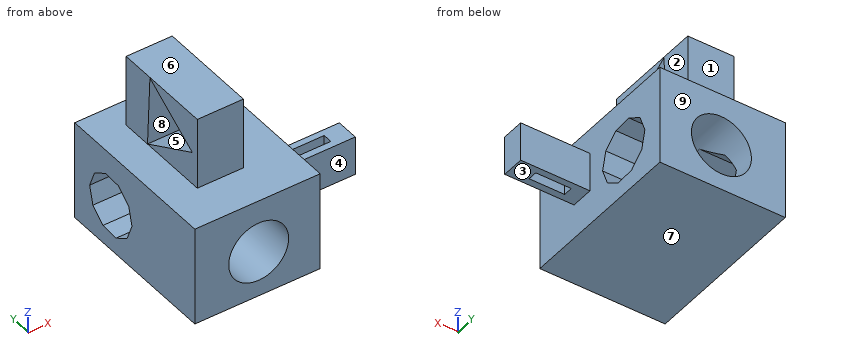
```python
from build123d import *

# Parameters (mm, degrees)
F0_W      = 94.7674
F0_H      = 75.057
F1_DEPTH  = 64.262
F2_W      = 34.8323993385
F2_H      = 76.1452428997
F3_DEPTH  = 92.202
F4_W      = 17.0815913007
F4_H      = 29.5642912388
F5_DEPTH  = 111.506
F6_W      = 26.8206745386
F6_H      = 7.122894749
F7_DEPTH  = 117.3734
F8_R      = 22.6565007862
F9_DEPTH  = 114.554
F11_DEPTH = 73.406
F13_DEPTH = 151.384


with BuildPart() as f1:
    # F0 (on Front) → F1 (new body, symmetric)
    with BuildSketch(Plane.XZ):
        with Locations((11.7503735555, 0.2659336123)):
            Rectangle(F0_W, F0_H)
    extrude(amount=F1_DEPTH, both=True)

    # F2 (on Top) → F3 (join)
    with BuildSketch(Plane.XY):
        with Locations((6.345430389, 5.9404056519)):
            Rectangle(F2_W, F2_H)
    extrude(amount=F3_DEPTH)

    # F4 (on Right) → F5 (join)
    with BuildSketch(Plane.YZ):
        with Locations((-19.0525432117, 3.8324072957)):
            Rectangle(F4_W, F4_H)
    extrude(amount=F5_DEPTH)

    # F6 (on face) → F7 (cut)
    with BuildSketch(Plane.XY.offset(18.6145529151)):
        with Locations((83.2830891013, -18.9009504393)):
            Rectangle(F6_W, F6_H)
    extrude(amount=-F7_DEPTH, mode=Mode.SUBTRACT)

    # F8 (on Front) → F9 (cut, symmetric)
    with BuildSketch(Plane.XZ):
        with Locations((12.634399347, -2.3397030309)):
            Circle(F8_R)
    extrude(amount=F9_DEPTH, both=True, mode=Mode.SUBTRACT)

    # F10 (on face) → F11 (cut, symmetric)
    with BuildSketch(Plane.YZ.offset(23.7616300583)):
        Polygon((18.5735931468, 91.7536235383), (-26.8142361042, 62.575721092), (21.1484832689, 37.8576591611), align=None)
    extrude(amount=F11_DEPTH, both=True, mode=Mode.SUBTRACT)

    # F12 (on face) → F13 (cut)
    with BuildSketch(Plane(origin=(-35.6333264445, 0, 0), x_dir=(0, -1, 0), z_dir=(-1, 0, 0))):
        Polygon((-2.9979522495, -4.1226996567), (-6.4409147017, 9.4672488049), (-17.2143011216, 18.4380255093), (-31.2030440708, 19.3630986611), (-43.0639192026, 11.8891217583), (-48.2664753528, -1.1291000534), (-44.8235129006, -14.719048515), (-34.0501264807, -23.6898252194), (-20.0613835315, -24.6148983712), (-8.2005083997, -17.1409214684), align=None)
    extrude(amount=-F13_DEPTH, mode=Mode.SUBTRACT)


solid = f1.part
```
Build history of the part. All positions in model axes, mm. Face numbers are marked on the shaded views. A direction names the side the tool comes from. Round coordinates to 2 decimals unless told otherwise and drop trailing zeros. Write each loop counter-clockwise with the first axis right and the second up, starting at its lowest first coordinate (ties: lowest second). Pieces come first, ordered by that corner, then holes.
1) Drill centre lines: probe 1 along X at (y, z) = (-51, -14.5); probe 2 along Z at (x, y) = (29, 43); probe 3 along X at (y, z) = (-6.5, 14). Where is each one in solid material? Low to high.
2) Band-saw the part on D-D, the plane x = 52.5. List the corners of the cut face in (y, z), and give its area (3 significant figures).
3) Band-saw the part on A-A, the plane x = 93. List the corners of the cut face in (y, z), and give its area (3 significant figures).
4) Band-saw the part on C-C, the plane z = 7. List the corners of the cut face in (x, y), and give its area (3 significant figures).
5) Band-saw the part on B-B, the plane y = 25. List the corners of the cut face in (x, z).
6) Pin check, flat tips, straight feed: pin 1 (3 mm diameter, centred on y = -35.5, z = 76.5, fed in from -X); pin 2 (21.5 mm diameter, centred on x = 88, z = 7.5, fed in from +Y); pin 3 (8 mm diameter, centred on x = 80, z = 5, fed in from -Y); pin 4 (10 mm diameter, centred on y = 44.5, z = 58, fed in from -X). Stop position of each tip, or through.
7) Mould opens along Z. For the marked faces 6, 7, 8 and 9 say: +Z half, -Z half, draft (parallel to the pull), parting line (faces both ways), or undercut.
8) 3-axis set-ups, long thin cutter, end or side, ignore diameter. For the marked faces 1, 2, 3, 4 and 5: which of +Z, -Z, +X, -X, +Y, -Y reach the whole face in a straight line?
Ans:
1. probe 1: x = -35.63 to -6.48, 31.75 to 59.13
1. probe 2: z = -37.26 to -18.01, 13.33 to 37.79
1. probe 3: x = -35.63 to -3.06, 28.33 to 59.13
2. outline: (-64.26, -37.26) - (64.26, -37.26) - (64.26, 37.79) - (-64.26, 37.79) - close; hole (3, -4.12) - (8.2, -17.14) - (20.06, -24.61) - (34.05, -23.69) - (44.82, -14.72) - (48.27, -1.13) - (43.06, 11.89) - (31.2, 19.36) - (17.21, 18.44) - (6.44, 9.47) - close
2. area: 8,130 mm2
3. outline: (-27.59, -10.95) - (-22.46, -10.95) - (-22.46, 18.61) - (-27.59, 18.61) - close; (-15.34, -10.95) - (-10.51, -10.95) - (-10.51, 18.61) - (-15.34, 18.61) - close
3. area: 294 mm2
4. outline: (-35.63, -64.26) - (-8.01, -64.26) - (-8.01, 5.82) - (-35.63, 5.82) - close; (-35.63, 45.02) - (-8.01, 45.02) - (-8.01, 64.26) - (-35.63, 64.26) - close; (33.28, -64.26) - (59.13, -64.26) - (59.13, -27.59) - (111.51, -27.59) - (111.51, -10.51) - (59.13, -10.51) - (59.13, 5.82) - (33.28, 5.82) - close; (33.28, 45.02) - (59.13, 45.02) - (59.13, 64.26) - (33.28, 64.26) - close; hole (69.87, -22.46) - (96.69, -22.46) - (96.69, -15.34) - (69.87, -15.34) - close
4. area: 5,480 mm2
5. outline: (-35.63, -37.26) - (59.13, -37.26) - (59.13, -24.29) - (18.25, -24.29) arc R22.66 cw to (7.02, -24.29) - (-35.63, -24.29) - close; (-35.63, 18.95) - (4.89, 18.95) arc R22.66 cw to (20.38, 18.95) - (59.13, 18.95) - (59.13, 37.79) - (23.76, 37.79) - (23.76, 92.2) - (-11.07, 92.2) - (-11.07, 37.79) - (-35.63, 37.79) - close
6. pin 1: passes through
6. pin 2: stops at y = -10.51
6. pin 3: stops at y = -27.59
6. pin 4: stops at x = -11.07
7. face 6: +Z half
7. face 7: -Z half
7. face 8: undercut
7. face 9: draft
8. face 1: +Z, +X, -X, +Y
8. face 2: +Z, +X, +Y, -Y
8. face 3: -Z, +X, +Y, -Y
8. face 4: +Z, -Z, +X, -Y
8. face 5: +X, -X
